Model file for the job. Use its own axes, mm. A direction names the side the tool comes from. Round coordinates to 2 decimals unless told otherwise and drop trailing zeros. Order: outer loops, then holes, each group sorted by start corner. A loop starts at its lowest first (then second) coordinate and runs counter-clockwise, first axis right, second up. Notation, with made-up numbers: (63.25, 31) - (102.25, 31) arc R23 ccw to (102.25, 48) - close; hole circle Ø11 at (87, -33). An arc over 180 degrees is marked (long way). Answer as CSV lines item,"result". Start each with the question number.
1. Band-saw the part on C-C on y = 13.25. List the corners of the cut face in (x, z), then the cut area to 3 significant figures.
2. Band-saw the part on B-B on x = 0. List the corners of the cut face in (y, z) (3 decimals).
3. Pin check, flat tips, straight feed: pin 1 Ø13 at (x, z) = (-1.5, -1.5) entering from -Y; pin 2 Ø10 at (x, z) = (0, -0.5) entering from +Y; pin 3 Ø0.9 at (x, z) = (-53, 17) entering from +Y. Stop position of each tip, or through.
4. 3-axis set-ups, long thin cutter, end or side, ignore diameter. For faces 1 (the face through (-16, 0, 0)), 2 (the face through (-51, -4, 14)), 3 (the face through (-51, -10, -18)): which of +Z, -Z, +X, -X, +Y, -Y reach the whole face in a straight line?
5. Band-saw the part on D-D on x = -33. List the corners of the cut face in (y, z).
6. Wall check: line 1 along Z through (x, y) = (0, 13.5); line 2 along X through (y, z) = (5.85, 0) (3 decimals); line 3 along X through (y, z) = (13, 0). Give the ranges that are in metal, low to high. Write a range as [from, to].
7. Band-saw the part on A-A on z = 0. List the corners of the cut face in (x, y) (3 decimals).
8. Pull direction Z, two halves, no side cores. Call faces 4 (the face through (-51, -10, 18)), 5 (the face through (0, 2.75, 0)), 6 (the face through (-26, 2, -4.75)): released by +Z, released by -Z, zero draft, split by the parting line, or undercut.
```python
from build123d import *

# Parameters (mm, degrees)
F_0_1MM_FIT_FOR_POT_R   = 10.5
BOSS_EXTRUDE1_DEPTH     = 2.75
SKETCH4_R               = 10.5
SKETCH4_R_2             = 8.275
BOSS_EXTRUDE2_DEPTH     = 4.25
BOSS_EXTRUDE3_DEPTH     = 2
FILLET1_R               = 0.25
BOSS_EXTRUDE6_DEPTH     = 10
BOSS_EXTRUDE7_DEPTH     = 2.9
BOSS_EXTRUDE8_DEPTH     = 3
FILLET2_R               = 1.5
BOSS_EXTRUDE9_DEPTH     = 17.5
SKETCH12_W              = 12.5
SKETCH12_H              = 6
CUT_EXTRUDE2_DEPTH      = 67.52567968
CUT_EXTRUDE2_DEPTH_BACK = 67.52567968


with BuildPart() as part:
    # 0.1mm fit for pot → Boss-Extrude1 (new body)
    with BuildSketch(Plane(origin=(0, 0, 0), x_dir=(1, 0, 0), z_dir=(0, 1, 0))):
        with Locations(Location((0, 0, 0), (0, 0, 270))):
            Circle(F_0_1MM_FIT_FOR_POT_R)
    extrude(amount=BOSS_EXTRUDE1_DEPTH)

    # Sketch4 → Boss-Extrude2 (add)
    with BuildSketch(Plane(origin=(0, 2.75, 0), x_dir=(1, 0, 0), z_dir=(0, 1, 0))):
        with Locations(Location((0, 0, 0), (0, 0, 270))):
            Circle(SKETCH4_R)
        with Locations(Location((0, 0, 0), (0, 0, 270))):
            Circle(SKETCH4_R_2, mode=Mode.SUBTRACT)
    extrude(amount=BOSS_EXTRUDE2_DEPTH)

    # Sketch5 → Boss-Extrude3 (add)
    with BuildSketch(Plane(origin=(0, 2.75, 0), x_dir=(1, 0, 0), z_dir=(0, 1, 0))):
        with BuildLine():
            Line((-1, -8.214354813), (-1, -7.065799598))
            Line((-1, -7.065799598), (0.988059701, -7.065799598))
            Line((0.988059701, -7.065799598), (0.988059701, -8.215799598))
            ThreePointArc((0.988059701, -8.215799598), (-0.006013695, -8.274997815), (-1, -8.214354813))
        make_face()
    extrude(amount=BOSS_EXTRUDE3_DEPTH)

    # Fillet1
    fillet1_edges = [part.edges().sort_by_distance(p)[0] for p in [
        (0.988059701, 3.75, 7.065799598),
        (-1, 3.75, 7.065799598),
        (-0.005970149, 4.75, 7.065799598),
        (-1, 4.75, 7.640077205),
        (0.988059701, 4.75, 7.640799598),
    ]]
    fillet(fillet1_edges, radius=FILLET1_R)

    # Sketch7 → Boss-Extrude6 (add)
    with BuildSketch(Plane(origin=(0, 7, 0), x_dir=(1, 0, 0), z_dir=(0, 1, 0))):
        with BuildLine():
            Line((3.299602194, 9.968080325), (3.299602194, 8.373328213))
            ThreePointArc((3.299602194, 8.373328213), (-9, 0), (3.299602194, -8.373328213))
            Line((3.299602194, -8.373328213), (3.299602194, -9.968080325))
            ThreePointArc((3.299602194, -9.968080325), (-10.5, 0), (3.299602194, 9.968080325))
        make_face()
    extrude(amount=BOSS_EXTRUDE6_DEPTH)

    # Sketch8 → Boss-Extrude7 (add)
    with BuildSketch(Plane(origin=(0, 17, 0), x_dir=(1, 0, 0), z_dir=(0, 1, 0))):
        with BuildLine():
            Line((3.299602194, 12.315645552), (3.299602194, 9.968080325))
            ThreePointArc((3.299602194, 9.968080325), (-10.5, 0), (3.299602194, -9.968080325))
            Line((3.299602194, -9.968080325), (3.299602194, -12.315645552))
            ThreePointArc((3.299602194, -12.315645552), (-12.75, 0), (3.299602194, 12.315645552))
        make_face()
    extrude(amount=-BOSS_EXTRUDE7_DEPTH)

    # Sketch9 → Boss-Extrude8 (add)
    with BuildSketch(Plane.XZ):
        with BuildLine():
            Line((-9.3641604, 4.75), (-59.3641604, 4.75))
            Line((-59.3641604, 4.75), (-59.3641604, -4.75))
            Line((-59.3641604, -4.75), (-9.3641604, -4.75))
            ThreePointArc((-9.3641604, -4.75), (-10.5, 0), (-9.3641604, 4.75))
        make_face()
    extrude(amount=-BOSS_EXTRUDE8_DEPTH)

    # Fillet2
    fillet2_edges = [part.edges().sort_by_distance(p)[0] for p in [
        (-10.5, 3, 0),
        (-9.3641604, 1.5, 4.75),
        (-9.3641604, 1.5, -4.75),
    ]]
    fillet(fillet2_edges, radius=FILLET2_R)

    # Sketch10 → Boss-Extrude9 (add)
    with BuildSketch(Plane.ZY.offset(59.3641604)):
        with BuildLine():
            Line((-20, -12), (-17, -12))
            add(Edge.make_bspline(
                [(-17, -12), (-13.13473835, -2.13897718), (-4.75, 0)],
                knots=[0, 0, 0, 0.391543848, 0.391543848, 0.391543848], degree=2))
            Line((-4.75, 0), (4.75, 0))
            add(Edge.make_bspline(
                [(4.75, 0), (13.134738349, -2.13897718), (17, -12)],
                knots=[0.608456152, 0.608456152, 0.608456152, 1, 1, 1], degree=2))
            Line((17, -12), (20, -12))
            add(Edge.make_bspline(
                [(4.75, 3), (15.273777711, 0.693481354), (20, -12)],
                knots=[0.590854454, 0.590854454, 0.590854454, 1, 1, 1], degree=2))
            Line((4.75, 3), (-4.75, 3))
            add(Edge.make_bspline(
                [(-20, -12), (-15.273777711, 0.693481354), (-4.75, 3)],
                knots=[0, 0, 0, 0.409145546, 0.409145546, 0.409145546], degree=2))
        make_face()
    extrude(amount=-BOSS_EXTRUDE9_DEPTH)

    # Sketch12 → Cut-Extrude2 (cut, two sides)
    with BuildSketch(Plane(origin=(0, 0, -4.75), x_dir=(-1, 0, 0), z_dir=(0, 0, -1))) as cut_extrude2_sk:
        with Locations((50.6141604, -7)):
            Rectangle(SKETCH12_W, SKETCH12_H)
    extrude(amount=CUT_EXTRUDE2_DEPTH, mode=Mode.SUBTRACT)
    extrude(cut_extrude2_sk.sketch, amount=-CUT_EXTRUDE2_DEPTH_BACK, mode=Mode.SUBTRACT)


solid = part.part
```
Reply:
1,outline,"(3.3, -9.97) - (3.3, -8.37) arc R9 cw (long way) to (3.3, 8.37) - (3.3, 9.97) arc R10.5 ccw (long way) to start"
1,area,"56.0 mm2"
2,outline,"(0, -10.5) - (14.1, -10.5) - (14.1, -12.75) - (17, -12.75) - (17, -9) - (7, -9) - (7, -8.275) - (2.75, -8.275) - (2.75, 7.066) - (4.5, 7.066) arc R0.25 ccw to (4.75, 7.316) - (4.75, 8.275) - (7, 8.275) - (7, 9) - (17, 9) - (17, 12.75) - (14.1, 12.75) - (14.1, 10.5) - (0, 10.5) - close"
3,pin 1,"stops at y = 0"
3,pin 2,"stops at y = 2.75"
3,pin 3,"stops at y = -10"
4,face 1,"+X, -Y"
4,face 2,"+Z, -Z, -Y"
4,face 3,"+Z, -Z, +Y"
5,outline,"(0, -4.75) - (3, -4.75) - (3, 4.75) - (0, 4.75) - close"
6,line 1,"z = [-10.5, -9], [9, 10.5]"
6,line 2,"x = [-10.5, -8.275], [8.275, 10.5]"
6,line 3,"x = [-10.5, -9]"
7,outline,"(-59.364, 0) - (10.5, 0) - (10.5, 7) - (8.275, 7) - (8.275, 2.75) - (-8.275, 2.75) - (-8.275, 7) - (-9, 7) - (-9, 17) - (-12.75, 17) - (-12.75, 14.1) - (-10.5, 14.1) - (-10.5, 4.5) arc R1.5 cw to (-12, 3) - (-59.364, 3) - close"
8,face 4,"zero draft"
8,face 5,"undercut"
8,face 6,"released by -Z"
